Source: CAD feature listing. Evaluate the final solid. Frame: model axes, mm. A direction names the side the tool comes from. Round coordinates to 2 decimals unless told otherwise and drop trailing zeros. Order: outer loops, then holes, each group sorted by start corner. A loop starts at its lowest first (then second) coordinate and runs counter-clockwise, first axis right, second up. Notation, with made-up numbers: M -24.75,-24.5 L -16.75,-24.5 A19 ccw -16.75,-18.5 Z; hole C 17,18 d1. An arc over 180 degrees is marked long. Answer as CSV lines item,"result". Start each with the question number.
Item 1: First-contact query: P1, Ø0.6, axis at y = 34, z = -1.5, coming from the -X side; P2, Ø0.6, axis at x = 50.5, y = 30, coming from the -Z side. Flat tips, straight axial feed; report the tip coordinate or a pass-through.
Item 2: Line query: line 1 (Y direction, x = 53, z = -16); line 2 (Y direction, x = 52.2, z = -6); line 3 (X direction, y = 36, z = -27). Output: solid intervals per line, ascending. Write a range as [from, to].
Item 3: Section query C-C on z = -19.5. Return the cut outline in (x, y), plus the area to 3 significant figures.
Item 4: Section query A-A on x = 54.3. Return the cut outline in (y, z), plus the area to 3 significant figures.
Item 5: Section query B-B on y = 6. Return the cut outline in (x, z), plus the area to 3 significant figures.
Item 6: Pull-direction query (Y, two-part tool) for faces 4 (the face through (52, 0, -16)), 5 (the face through (50.6, 10, -15.5)); classes: +Y half, -Y half, draft (parallel to the pull), parting line (faces both ways), or undercut.
Item 7: Set-up query: faces 1 (the face through (52.54, 4.94, -24.61)), 2 (the face through (50.6, 10, -31.5)), 3 (the face through (51, 27, -8.9)). Return all of +Z, -Z, +X, -X, +Y, -Y with unobstructed straight access to the full face (end or side cutting, diameter ignored); none if empty.
from build123d import *

# Parameters (mm, degrees)
SKETCH1_W           = 55
SKETCH1_H           = 32
BOSS_EXTRUDE1_DEPTH = 46
SKETCH2_W           = 45
SKETCH2_H           = 32
CUT_EXTRUDE1_DEPTH  = 45
SKETCH3_R           = 1.75
CUT_EXTRUDE2_DEPTH  = 47
SKETCH4_R           = 1.75
CUT_EXTRUDE3_DEPTH  = 56
SKETCH5_W           = 1.1
SKETCH5_H           = 35
CUT_EXTRUDE4_DEPTH  = 1.2
SKETCH7_W           = 32
SKETCH7_H           = 46
CUT_EXTRUDE5_DEPTH  = 50


with BuildPart() as part:
    # Sketch1 → Boss-Extrude1 (new body)
    with BuildSketch(Plane(origin=(0, 0, 0), x_dir=(1, 0, 0), z_dir=(0, 1, 0))):
        with Locations((27.5, 16)):
            Rectangle(SKETCH1_W, SKETCH1_H)
    extrude(amount=BOSS_EXTRUDE1_DEPTH)

    # Sketch2 → Cut-Extrude1 (cut)
    with BuildSketch(Plane.XZ):
        with Locations((27.5, -16)):
            Rectangle(SKETCH2_W, SKETCH2_H)
    extrude(amount=-CUT_EXTRUDE1_DEPTH, mode=Mode.SUBTRACT)

    # Sketch3 → Cut-Extrude2 (cut, through all)
    with BuildSketch(Plane(origin=(0, 46, 0), x_dir=(1, 0, 0), z_dir=(0, 1, 0))):
        with Locations((43.5, 26)):
            Circle(SKETCH3_R)
        with Locations((43.5, 6)):
            Circle(SKETCH3_R)
        with Locations((11.5, 26)):
            Circle(SKETCH3_R)
        with Locations((11.5, 6)):
            Circle(SKETCH3_R)
    extrude(amount=-CUT_EXTRUDE2_DEPTH, mode=Mode.SUBTRACT)

    # Sketch4 → Cut-Extrude3 (cut, through all)
    with BuildSketch(Plane(origin=(55, 0, 0), x_dir=(0, 0, -1), z_dir=(1, 0, 0))):
        with Locations((6, 6)):
            Circle(SKETCH4_R)
        with Locations((26, 6)):
            Circle(SKETCH4_R)
        with Locations((16, 42)):
            Circle(SKETCH4_R)
    extrude(amount=-CUT_EXTRUDE3_DEPTH, mode=Mode.SUBTRACT)

    # Sketch5 → Cut-Extrude4 (cut)
    with BuildSketch(Plane.ZY.offset(-50)):
        with Locations((-29.45, 27.5)):
            Rectangle(SKETCH5_W, SKETCH5_H)
        with Locations((-31.45, 27.5)):
            Rectangle(SKETCH5_W, SKETCH5_H)
        with Locations((-27.45, 27.5)):
            Rectangle(SKETCH5_W, SKETCH5_H)
        with Locations((-25.45, 27.5)):
            Rectangle(SKETCH5_W, SKETCH5_H)
        with Locations((-23.45, 27.5)):
            Rectangle(SKETCH5_W, SKETCH5_H)
        with Locations((-21.45, 27.5)):
            Rectangle(SKETCH5_W, SKETCH5_H)
        with Locations((-19.45, 27.5)):
            Rectangle(SKETCH5_W, SKETCH5_H)
        with Locations((-17.45, 27.5)):
            Rectangle(SKETCH5_W, SKETCH5_H)
        with Locations((-15.45, 27.5)):
            Rectangle(SKETCH5_W, SKETCH5_H)
        with Locations((-13.45, 27.5)):
            Rectangle(SKETCH5_W, SKETCH5_H)
        with Locations((-11.45, 27.5)):
            Rectangle(SKETCH5_W, SKETCH5_H)
        with Locations((-9.45, 27.5)):
            Rectangle(SKETCH5_W, SKETCH5_H)
        with Locations((-7.45, 27.5)):
            Rectangle(SKETCH5_W, SKETCH5_H)
        with Locations((-5.45, 27.5)):
            Rectangle(SKETCH5_W, SKETCH5_H)
        with Locations((-3.45, 27.5)):
            Rectangle(SKETCH5_W, SKETCH5_H)
        with Locations((-1.45, 27.5)):
            Rectangle(SKETCH5_W, SKETCH5_H)
        with Locations((0.55, 27.5)):
            Rectangle(SKETCH5_W, SKETCH5_H)
    extrude(amount=-CUT_EXTRUDE4_DEPTH, mode=Mode.SUBTRACT)

    # Sketch7 → Cut-Extrude5 (cut)
    with BuildSketch(Plane.ZY):
        with Locations((-16, 23)):
            Rectangle(SKETCH7_W, SKETCH7_H)
    extrude(amount=-CUT_EXTRUDE5_DEPTH, mode=Mode.SUBTRACT)


solid = part.part
Results:
1,P1,"x = 51.2"
1,P2,"z = -30.9"
2,line 1,"[0, 40.25], [43.75, 46]"
2,line 2,"[0, 4.25], [7.75, 46]"
2,line 3,"[51.2, 55]"
3,outline,"M 50,0 L 55,0 L 55,46 L 50,46 L 50,45 L 51.2,45 L 51.2,10 L 50,10 Z"
3,area,"188 mm^2"
4,outline,"M 0,-32 L 46,-32 L 46,0 L 0,0 Z; hole C 6,-26 d3.5; hole C 6,-6 d3.5; hole C 42,-16 d3.5"
4,area,"1,440 mm^2"
5,outline,"M 50,-32 L 55,-32 L 55,-27.75 L 50,-27.75 Z; M 50,-24.25 L 55,-24.25 L 55,-7.75 L 50,-7.75 Z; M 50,-4.25 L 55,-4.25 L 55,0 L 50,0 Z"
5,area,"125 mm^2"
6,face 4,"-Y half"
6,face 5,"undercut"
7,face 1,"+X, -X"
7,face 2,"-Z, -X"
7,face 3,"-X"
